Could you check a few things on this model? Use its own coordinates, in mm. A direction names the side the tool comes from. Coordinates: 2 decimals unless noted, no trailing zeros. Order: outer loops, then holes, each group sorted by start corner. A loop starts at its lowest first (then second) coordinate and runs counter-clockwise, first axis right, second up. Notation, with made-up numbers: (49, 59.5) -> (88, 59.5) arc R7 ccw to (88, 66.5) -> close; hole circle Ø6 at (20, 76.5). An arc over 180 degrees is marked (long way). Return JSON: item names as keys, results as strings. Group by question number.
from build123d import *

# Parameters (mm, degrees)
F0_W      = 170
F0_H      = 76
F0_W_2    = 164
F0_H_2    = 70
F1_DEPTH  = 3
F2_DEPTH  = 40
F4_DEPTH  = 35.9
F5_DEPTH  = 36.4
F6_R      = 1.4
F7_DEPTH  = 0.5
F9_R      = 1.4
F10_DEPTH = 0.5
F12_R     = 5
F13_W     = 5
F13_H     = 60
F14_DEPTH = 5
F15_R     = 1


# Not quite as in the source:
# - a fillet or chamfer that OpenCascade refuses, or shapes differently, is made with other operations: its cross-section is extruded or revolved along the edge and cut away or added


with BuildPart() as f1:
    # F0 (on Top) → F1 (new body)
    with BuildSketch(Plane.XY):
        Rectangle(F0_W, F0_H)
        Rectangle(F0_W_2, F0_H_2, mode=Mode.SUBTRACT)
        Rectangle(F0_W_2, F0_H_2)
    extrude(amount=-F1_DEPTH)

    # F0 (on Top) → F2 (join)
    with BuildSketch(Plane.XY):
        Rectangle(F0_W, F0_H)
        Rectangle(F0_W_2, F0_H_2, mode=Mode.SUBTRACT)
    extrude(amount=F2_DEPTH)

    # F3 (on Front) → F4 (join, symmetric)
    with BuildSketch(Plane.XZ):
        Polygon((-82, 11), (-82, 9), (-71, 9), (0, 9), (5.6, 9), (38, 9), (38, 11), align=None)
    extrude(amount=F4_DEPTH, both=True)

    # F3 (on Front) → F5 (join, symmetric)
    with BuildSketch(Plane.XZ):
        Polygon((-82, 22), (-82, 20), (-71, 20), (5.6, 20), (38, 20), (38, 22), align=None)
    extrude(amount=F5_DEPTH, both=True)

    # F6 (on face) → F7 (join)
    with BuildSketch(Plane.XZ.offset(-35)):
        with Locations((-71, 16)):
            Circle(F6_R)
        with Locations((-71, 5)):
            Circle(F6_R)
        with Locations((5.6, 5)):
            Circle(F6_R)
        with Locations((5.6, 16)):
            Circle(F6_R)
    extrude(amount=F7_DEPTH)

    # F8: fillet of radius 1 on 4 edges, made by hand

    # F8_s1 → F8_t2 (revolve, cut)
    with BuildSketch(Plane.XY.offset(16)):
        with BuildLine():
            ThreePointArc((-69.6, 35), (-69.9660254038, 34.6339745962), (-70.4660254038, 34.5))
            Line((-70.4660254038, 34.5), (-69.6, 34.5))
            Line((-69.6, 34.5), (-69.6, 35))
        make_face()
    revolve(axis=Axis((-71, 34.5, 16), (0, -1, 0)), mode=Mode.SUBTRACT)

    # F8_s3 → F8_t4 (revolve, cut)
    with BuildSketch(Plane.XY.offset(5)):
        with BuildLine():
            ThreePointArc((-69.6, 35), (-69.9660254038, 34.6339745962), (-70.4660254038, 34.5))
            Line((-70.4660254038, 34.5), (-69.6, 34.5))
            Line((-69.6, 34.5), (-69.6, 35))
        make_face()
    revolve(axis=Axis((-71, 34.5, 5), (0, -1, 0)), mode=Mode.SUBTRACT)

    # F8_s5 → F8_t6 (revolve, cut)
    with BuildSketch(Plane.XY.offset(16)):
        with BuildLine():
            ThreePointArc((7, 35), (6.6339745962, 34.6339745962), (6.1339745962, 34.5))
            Line((6.1339745962, 34.5), (7, 34.5))
            Line((7, 34.5), (7, 35))
        make_face()
    revolve(axis=Axis((5.6, 34.5, 16), (0, -1, 0)), mode=Mode.SUBTRACT)

    # F8_s7 → F8_t8 (revolve, cut)
    with BuildSketch(Plane.XY.offset(5)):
        with BuildLine():
            ThreePointArc((7, 35), (6.6339745962, 34.6339745962), (6.1339745962, 34.5))
            Line((6.1339745962, 34.5), (7, 34.5))
            Line((7, 34.5), (7, 35))
        make_face()
    revolve(axis=Axis((5.6, 34.5, 5), (0, -1, 0)), mode=Mode.SUBTRACT)

    # F9 (on face) → F10 (join)
    with BuildSketch(Plane(origin=(0, -35, 0), x_dir=(-1, 0, 0), z_dir=(0, 1, 0))):
        with Locations((71, 16)):
            Circle(F9_R)
        with Locations((-5.6, 16)):
            Circle(F9_R)
        with Locations((-5.6, 5)):
            Circle(F9_R)
        with Locations((71, 5)):
            Circle(F9_R)
    extrude(amount=F10_DEPTH)

    # F11: fillet of radius 1 on 4 edges, made by hand

    # F11_s1 → F11_t2 (revolve, cut)
    with BuildSketch(Plane.XY.offset(16)):
        with BuildLine():
            ThreePointArc((-72.4, -35), (-72.0339745962, -34.6339745962), (-71.5339745962, -34.5))
            Line((-71.5339745962, -34.5), (-72.4, -34.5))
            Line((-72.4, -34.5), (-72.4, -35))
        make_face()
    revolve(axis=Axis((-71, -34.5, 16), (0, 1, 0)), mode=Mode.SUBTRACT)

    # F11_s3 → F11_t4 (revolve, cut)
    with BuildSketch(Plane.XY.offset(5)):
        with BuildLine():
            ThreePointArc((-72.4, -35), (-72.0339745962, -34.6339745962), (-71.5339745962, -34.5))
            Line((-71.5339745962, -34.5), (-72.4, -34.5))
            Line((-72.4, -34.5), (-72.4, -35))
        make_face()
    revolve(axis=Axis((-71, -34.5, 5), (0, 1, 0)), mode=Mode.SUBTRACT)

    # F11_s5 → F11_t6 (revolve, cut)
    with BuildSketch(Plane.XY.offset(16)):
        with BuildLine():
            ThreePointArc((4.2, -35), (4.5660254038, -34.6339745962), (5.0660254038, -34.5))
            Line((5.0660254038, -34.5), (4.2, -34.5))
            Line((4.2, -34.5), (4.2, -35))
        make_face()
    revolve(axis=Axis((5.6, -34.5, 16), (0, 1, 0)), mode=Mode.SUBTRACT)

    # F11_s7 → F11_t8 (revolve, cut)
    with BuildSketch(Plane.XY.offset(5)):
        with BuildLine():
            ThreePointArc((4.2, -35), (4.5660254038, -34.6339745962), (5.0660254038, -34.5))
            Line((5.0660254038, -34.5), (4.2, -34.5))
            Line((4.2, -34.5), (4.2, -35))
        make_face()
    revolve(axis=Axis((5.6, -34.5, 5), (0, 1, 0)), mode=Mode.SUBTRACT)

    # F12
    f12_edges = [f1.edges().sort_by_distance(p)[0] for p in [
        (-85, 38, 18.5),
        (-85, -38, 18.5),
        (-85, 0, -3),
        (0, 38, -3),
        (0, -38, -3),
    ]]
    fillet(f12_edges, radius=F12_R)

    # F13 (on face) → F14 (cut)
    with BuildSketch(Plane.XY):
        Rectangle(F13_W, F13_H)
    extrude(amount=-F14_DEPTH, mode=Mode.SUBTRACT)

    # F15
    f15_edges = [f1.edges().sort_by_distance(p)[0] for p in [
        (0, 30, 0),
        (-2.5, 30, -1.5),
        (0, 30, -3),
        (2.5, 30, -1.5),
        (0, -30, 0),
        (2.5, -30, -1.5),
        (0, -30, -3),
        (-2.5, -30, -1.5),
        (-2.5, 0, -3),
        (2.5, 0, -3),
        (-2.5, 0, 0),
        (2.5, 0, 0),
    ]]
    fillet(f15_edges, radius=F15_R)


solid = f1.part
Q1. I need wall thicknesses on line 1 along Z through (x, y) = (-12, 6); line 2 along X through (y, z) = (22.5, 25); line 3 along Y through (x, z) = (42, 32.5). Which ranges of each line are inside material? Lowest first, please. Write a range as from..to.
Q2. On a 3-axis mill with a long thin cutter (end or side, diameter ignored), from which of +Z, -Z, +X, -X, +Y, -Y can I reach the whole of each face in a straight line? I mean faces 1 (the flat face through (82, 0, 20)), 2 (the flat face through (20, 0, -3)), 3 (the flat face through (-19, 0, 0)). Say none if no direction works.
Q3. I'm going to push flat-ended pins straight in: pin 1 Ø0.5 at (x, z) = (0.5, -1.5) entering from -Y; pin 2 Ø21 at (x, y) = (-40.5, -7) entering from +Z. Where does each tip first touch, or does it pass through?
Q4. I want a section at C-C on z = 13. Please give me the cut outline in (x, y).
Q5. I want a section at B-B on x = -44.5. Please give me the cut outline in (y, z), and give its area (3 significant figures).
Q6. I want a section at D-D on x = 51. Please give me the cut outline in (y, z).
Q7. We'd pull the mould along Z, two halves only. Please class faces 4 (the flat face through (1, -38, 21)), 5 (the cylindrical face through (-84, 0, -1)), 6 (the flat face through (-82, 0, 15)): pulls with the +Z half, pulls with the -Z half, needs draft (parallel to the pull), parting line crosses it, or undercut.
Q8. I want a section at A-A on y = 9.5. Please give me the cut outline in (x, z).
Response values:
{
 "1": {"line 1": "z = -3..0, 9..11, 20..22", "line 2": "x = -85..-82, 82..85", "line 3": "y = -38..-35, 35..38"},
 "2": {"face 1": "+Z", "face 2": "-Z, +X, -X, +Y, -Y", "face 3": "none"},
 "3": {"pin 1": "stops at y = -36.8", "pin 2": "stops at z = 22"},
 "4": {"outline": "(-85, -33) arc R5 ccw to (-80, -38) -> (85, -38) -> (85, 38) -> (-80, 38) arc R5 ccw to (-85, 33) -> close; hole (-82, -35) -> (82, -35) -> (82, 35) -> (-82, 35) -> close"},
 "5": {"outline": "(-38, 2) arc R5 ccw to (-33, -3) -> (33, -3) arc R5 ccw to (38, 2) -> (38, 40) -> (35, 40) -> (35, 22) -> (-35, 22) -> (-35, 40) -> (-38, 40) -> close; hole (-35, 0) -> (35, 0) -> (35, 9) -> (-35, 9) -> close; hole (-35, 11) -> (35, 11) -> (35, 20) -> (-35, 20) -> close", "area": "737 mm²"},
 "6": {"outline": "(-38, 2) arc R5 ccw to (-33, -3) -> (33, -3) arc R5 ccw to (38, 2) -> (38, 40) -> (35, 40) -> (35, 0) -> (-35, 0) -> (-35, 40) -> (-38, 40) -> close"},
 "7": {"face 4": "needs draft", "face 5": "pulls with the -Z half", "face 6": "undercut"},
 "8": {"outline": "(-85, 2) arc R5 ccw to (-80, -3) -> (-3.5, -3) arc R1 ccw to (-2.5, -2) -> (-2.5, -1) arc R1 ccw to (-3.5, 0) -> (-82, 0) -> (-82, 9) -> (38, 9) -> (38, 11) -> (-82, 11) -> (-82, 20) -> (38, 20) -> (38, 22) -> (-82, 22) -> (-82, 40) -> (-85, 40) -> close; (2.5, -2) arc R1 ccw to (3.5, -3) -> (85, -3) -> (85, 40) -> (82, 40) -> (82, 0) -> (3.5, 0) arc R1 ccw to (2.5, -1) -> close"}
}
